Source: three-view drawing plus pictorial views. Frame: mm from the lowest corner of the part. A direction names the side the tool comes from. Round coordinates to 2 decimals unless told otherwise and drop trailing zeros. Loops run counter-clockwise (first coordinate to the right, second up) from the corner with the lowest first, then second, coordinate; pieces in that order, holes last. Notation, with made-up numbers: (-14, -33.75) -> (19, -33.75) arc R21 cw to (19, -26.75) -> close; hole circle Ø10 at (27, 15). An arc over 180 degrees is marked (long way). One line per question, with ' | ' between items. Start each with the question number.
Q1. Cut plane C-C on x = 59. Return loops of the section in (y, z).
Q2. Mould query, pull axis Z, two halves, no side actions, for the marked faces 1, 2 and 3. Classes: pulls with the +Z half, pulls with the -Z half, needs draft (parallel to the pull), parting line crosses it, or undercut.
Q3. Access query for the marked faces 4 and 5. Directions: +Z, -Z, +X, -X, +Y, -Y. A direction counts if a zero-diameter tool reaches every point of the face in a straight line with its end or side. Return the directions, or none.
Q4. Contact query for a flat-ended pin moving along its axis: P1, Ø6, axis at x = 27.5, z = 7, coming from the +Y side. Output: stop coordinate, or through.
Q5. Cut plane B-B on y = 212. Return loops of the section in (x, z).
Q6. Material intervals for L1, parallel to Z at x = 53.5, y = 205; L2, parallel to X at y = 139, z = 3.75, sorted ascending.
Q7. Cut plane A-A on z = 6.5. Return loops of the section in (x, y).
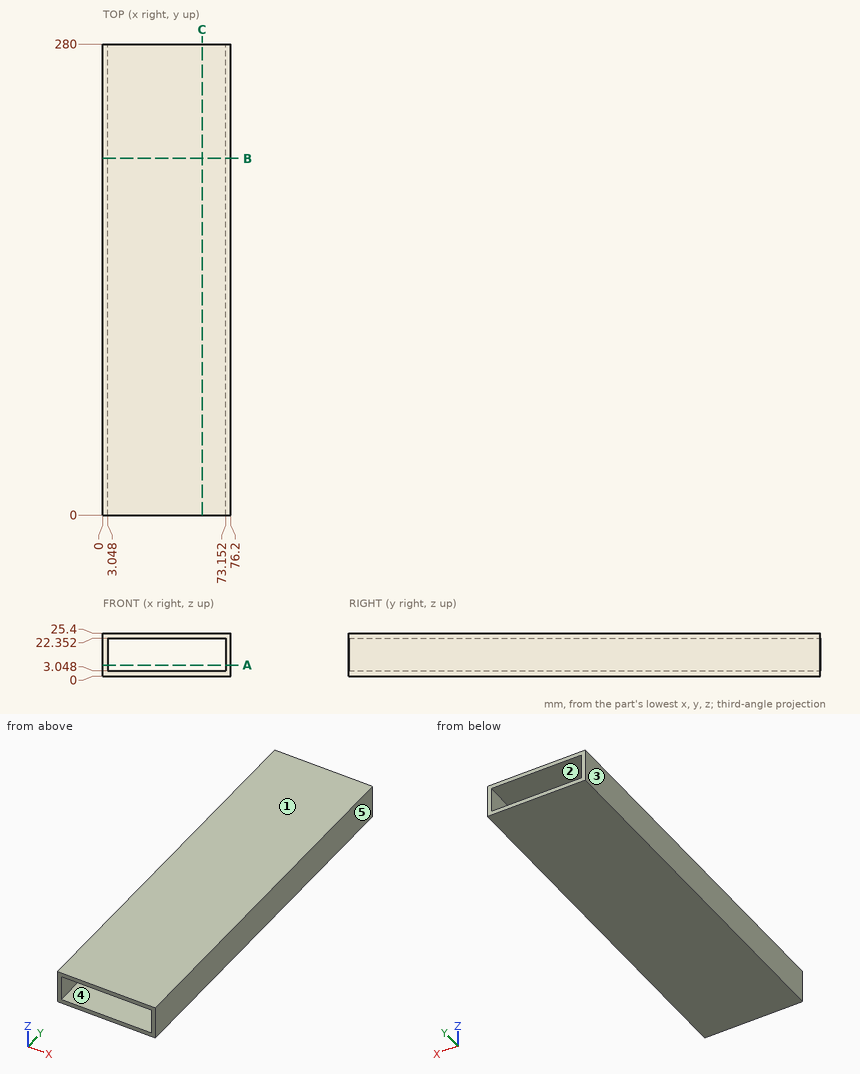
Results:
1) outline: (0, 0) -> (280, 0) -> (280, 3.05) -> (0, 3.05) -> close; (0, 22.35) -> (280, 22.35) -> (280, 25.4) -> (0, 25.4) -> close
2) face 1: pulls with the +Z half | face 2: undercut | face 3: needs draft
3) face 4: +Y, -Y | face 5: +Z, -Z, +X, +Y, -Y
4) P1: through
5) outline: (0, 0) -> (76.2, 0) -> (76.2, 25.4) -> (0, 25.4) -> close; hole (3.05, 3.05) -> (73.15, 3.05) -> (73.15, 22.35) -> (3.05, 22.35) -> close
6) L1: 0 to 3.05, 22.35 to 25.4 | L2: 0 to 3.05, 73.15 to 76.2
7) outline: (0, 0) -> (3.05, 0) -> (3.05, 280) -> (0, 280) -> close; (73.15, 0) -> (76.2, 0) -> (76.2, 280) -> (73.15, 280) -> close
